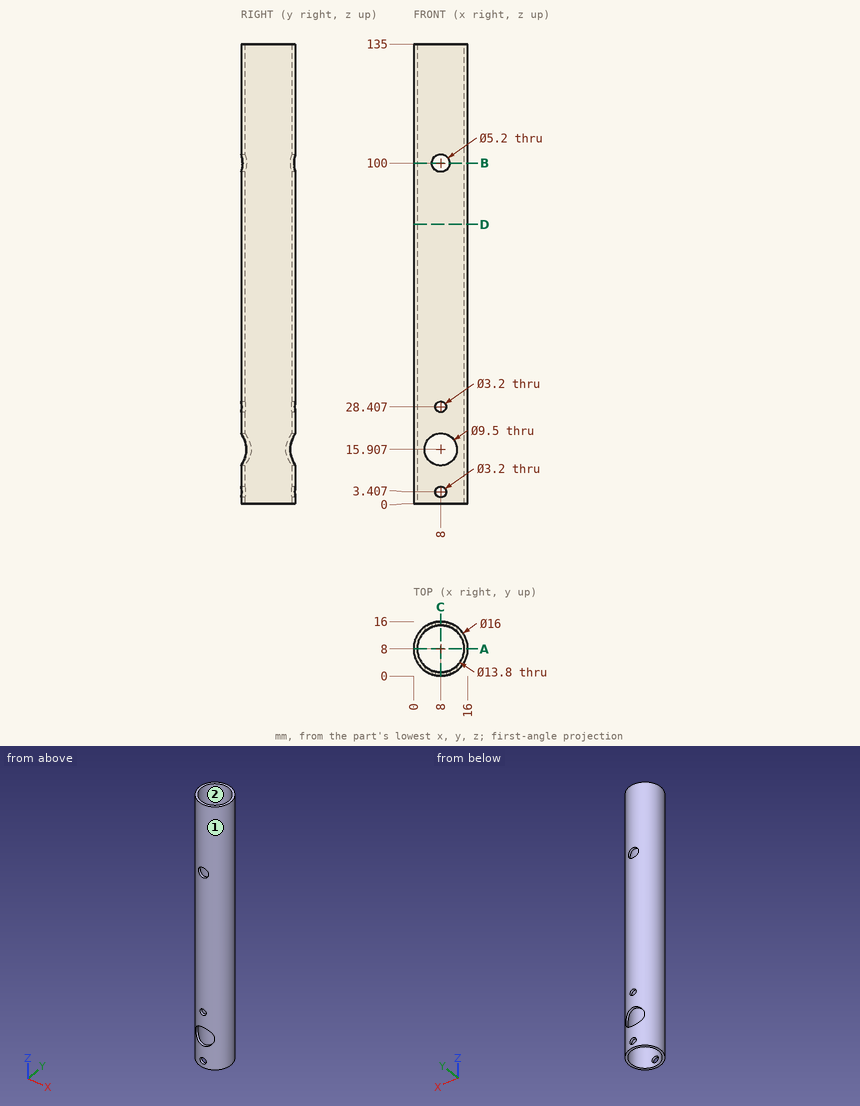
Design review of the part shown in the three views and the two pictorial views. Dimensions are in mm from the part's minimum x, y and z. Coordinates: 2 decimals unless noted, no trailing zeros. Loops run counter-clockwise (first coordinate to the right, second up) from the corner with the lowest first, then second, coordinate; pieces in that order, holes last.
(1) Insertion check: P1, Ø6, axis at x = 11.5, z = 66, coming from the -Y side; P2, Ø3, axis at x = 14, z = 118.5, coming from the -Y side; P3, Ø2, axis at y = 14, z = 41, coming from the +X side (3 decimals). Each pin has a flat end and moves straight along its axis. Give the tip position at first contact, or say it passes through.
Determined:
P1: stops at y = 0.02
P2: stops at y = 1.39
P3: stops at x = 14.245
(2) Consider section B-B, the plane z = 100. Give the boundary of the cut face in (x, y).
Determined:
outline: (5.4, 0.43) - (5.4, 1.61) arc R6.9 cw to (5.4, 14.39) - (5.4, 15.57) arc R8 ccw to start; (10.6, 0.43) arc R8 ccw to (10.6, 15.57) - (10.6, 14.39) arc R6.9 cw to (10.6, 1.61) - close
(3) Consider section C-C, the plane x = 8. Give the number of separate pieces and of enclosed holes in the cut face.
Determined:
separate pieces: 10
enclosed holes: 0
(4) Consider section D-D, the plane z = 82. Give the boundary of the cut face in (x, y), plus the area to 3 significant figures.
Determined:
outline: circle Ø16 at (8, 8); hole circle Ø13.8 at (8, 8)
area: 51.5 mm2
(5) Consider section A-A, the plane y = 8. Give the boundary of the cut face in (x, z), plus the area to 3 significant figures.
Determined:
outline: (0, 0) - (1.1, 0) - (1.1, 135) - (0, 135) - close; (14.9, 0) - (16, 0) - (16, 135) - (14.9, 135) - close
area: 297 mm2
(6) Draft analysis for pull direction X (two halves, no side actions). For the marked faces 1 and 2, state which applies: +X half, -X half, draft (parallel to the pull), parting line (faces both ways), or undercut.
Determined:
face 1: parting line
face 2: undercut
(7) Wall thickness on L1, parallel to X at y = 8.5, z = 42.5; L2, parallel to X at y = 12.25, z = 78: over which ranges is each line inside the solid? List them lowest first.
Determined:
L1: x = 0.02 to 1.12, 14.88 to 15.98
L2: x = 1.22 to 2.56, 13.44 to 14.78
